Read the model definition and answer for the solid it produces. Units are mm, in the model's axes. A direction names the side the tool comes from. Coordinates: 2 decimals unless noted, no trailing zeros. Order: outer loops, then holes, each group sorted by start corner. A loop starts at its lowest first (then second) coordinate and runs counter-clockwise, first axis right, second up.
from build123d import *

# Parameters (mm, degrees)
EXTRUDE_1_DEPTH = 70


with BuildPart() as part:
    # 草圖1 → 填料-伸長1 (new body)
    with BuildSketch(Plane(origin=(0, 0, 0), x_dir=(1, 0, 0), z_dir=(0, 1, 0))):
        with BuildLine():
            Line((10.996587269, 18.037741282), (-45.487838574, -38.61479297))
            ThreePointArc((-45.487838574, -38.61479297), (-47.84934361, -38.895811815), (-49.888582931, -37.672218494))
            Line((-49.888582931, -37.672218494), (-59.802776425, -27.787443971))
            Line((-59.802776425, -27.787443971), (-54.860389164, -22.830347224))
            Line((-54.860389164, -22.830347224), (-57.919724227, -19.780090306))
            Line((-57.919724227, -19.780090306), (-64.980277457, -26.861657088))
            Line((-64.980277457, -26.861657088), (-52.0067489, -39.796688528))
            ThreePointArc((-52.0067489, -39.796688528), (-47.849605549, -41.783872953), (-43.363368539, -40.732958939))
            Line((-43.363368539, -40.732958939), (13.121057303, 15.919575313))
            ThreePointArc((13.121057303, 15.919575313), (15.009846467, 17.808364477), (16.898635631, 15.919575313))
            Line((16.898635631, 15.919575313), (49.482242531, -40.323722611))
            ThreePointArc((49.482242531, -40.323722611), (54.046060411, -42.29505362), (58.903884757, -41.238586769))
            Line((58.903884757, -41.238586769), (73.314668888, -32.889941818))
            Line((73.314668888, -32.889941818), (69.304378808, -25.967689766))
            Line((69.304378808, -25.967689766), (67.007535769, -27.298327077))
            Line((67.007535769, -27.298327077), (69.513967069, -31.624734609))
            Line((69.513967069, -31.624734609), (57.400025977, -38.642742249))
            ThreePointArc((57.400025977, -38.642742249), (54.765652782, -39.530436118), (52.078087051, -38.819863831))
            Line((52.078087051, -38.819863831), (19.494480151, 17.423434093))
            ThreePointArc((19.494480151, 17.423434093), (15.47366289, 20.886366054), (10.996587269, 18.037741282))
        make_face()
    extrude(amount=EXTRUDE_1_DEPTH)


solid = part.part
Q1. The part is cut by section B-B, the plane z = 36. Determine the outline of the cut face in (x, y).
Q2. Straight lines are drawn through the part: L1, parallel to X at y = 63, z = 25; L2, parallel to X at y = 5, z = 37; L3, parallel to X at y = 49, z = 32.5. For each, find the intervals that lie inside material, in ascending order.
Q3. The part is cut by section C-C, the plane z = -13. Determine the outline of the cut face in (x, y), then the cut area to 3 significant figures.
Q4. The part is cut by section A-A, the plane y = 58.5. Determine the outline of the cut face in (x, z).
Q5. Which of the six approach directions +Z, -Z, +X, -X, +Y, -Y give full straight-line access (tool end or side, diameter ignored) to faces 5 (the flat face through (32.962, 34.51, 11.808)), 6 (the flat face through (-54.776, 34.51, 32.799)), 7 (the flat face through (-12, 0, 8)), 8 (the flat face through (-16.85, 34.51, 9.89)), 9 (the flat face through (-58.584, 34.51, 33.239))?
Q6. Each of these flat-tipped pins is pushed along its axis until it touches: P1, Ø2, axis at x = -46, y = 36, coming from the +Z side; P2, Ø6, axis at y = 61.5, z = 22.5, coming from the +X side; P3, Ø1.5, axis at y = 51, z = -14, coming from the -X side; P4, Ø10, axis at x = -39, z = 22.5, coming from the -Y side. Where does it stop, or does it pass through?
Q7. The part is cut by section D-D, the plane x = 29. Determine the outline of the cut face in (y, z).
Q8. Determine the mould class of faces 1 (the flat face through (-56.369, 34.51, 21.327)), 2 (the flat face through (71.34, 34.51, 29.48)), 3 (the flat face through (-61.4, 34.51, 23.27)), 4 (the cylindrical face through (15.55, 34.51, -20.88)) for opening direction X: +X half, -X half, draft (parallel to the pull), parting line (faces both ways), or undercut.
Computed values:
1. outline: (-55.81, 0) - (-51.57, 0) - (-51.57, 70) - (-55.81, 70) - close; (-42.88, 0) - (-38.64, 0) - (-38.64, 70) - (-42.88, 70) - close; (46.98, 0) - (50.44, 0) - (50.44, 70) - (46.98, 70) - close; (61.96, 0) - (67.95, 0) - (67.95, 70) - (61.96, 70) - close
2. L1: x = -63.12 to -57.02, -31.91 to -27.68, 40.6 to 44.07
2. L2: x = -54.81 to -50.56, -43.88 to -39.64, 47.56 to 51.02, 60.24 to 66.22
2. L3: x = -59.33 to -55.08, -39.39 to -35.15, 44.95 to 48.42, 68 to 73.09
3. outline: (5.97, 0) - (10.21, 0) - (10.21, 70) - (5.97, 70) - close; (18.59, 0) - (22.06, 0) - (22.06, 70) - (18.59, 70) - close
3. area: 539 mm2
4. outline: (-64.98, 26.86) - (-57.92, 19.78) - (-54.86, 22.83) - (-59.8, 27.79) - (-49.89, 37.67) arc R3.68 cw to (-45.49, 38.61) - (11, -18.04) arc R4.45 ccw to (19.49, -17.42) - (52.08, 38.82) arc R4.83 cw to (57.4, 38.64) - (69.51, 31.62) - (67.01, 27.3) - (69.3, 25.97) - (73.31, 32.89) - (58.9, 41.24) arc R8.12 ccw to (49.48, 40.32) - (16.9, -15.92) arc R1.89 cw to (13.12, -15.92) - (-43.36, 40.73) arc R6.95 ccw to (-52.01, 39.8) - close
5. face 5: +Z, +Y, -Y
5. face 6: +Y, -Y
5. face 7: +Z, -Z, +X, -X, -Y
5. face 8: -Z, +Y, -Y
5. face 9: +Z, -X, +Y, -Y
6. P1: stops at z = 41.82
6. P2: stops at x = 44.36
6. P3: stops at x = 6.22
6. P4: passes through
7. outline: (0, -1.02) - (70, -1.02) - (70, 4.97) - (0, 4.97) - close
8. face 1: undercut
8. face 2: +X half
8. face 3: -X half
8. face 4: parting line
